The model under review builds one solid part; all positions refer to its coordinate system, in mm. Face numbers are marked on the shaded views. A direction names the side the tool comes from. Round coordinates to 2 decimals unless told otherwise and drop trailing zeros. Order: outer loops, then holes, each group sorted by start corner. A loop starts at its lowest first (then second) coordinate and runs counter-clockwise, first axis right, second up.
1) Consider section C-C (x = 391). Give the boundary of the cut face in (y, z), then the cut area to 3 significant figures.
2) Machinability: for the marked faces 4 and 5, which of the approach directions +Z, -Z, +X, -X, +Y, -Y give a long, thin tool a straight path to every point of the face, cutting with its end or side? Answer none if there is none.
3) To check wall thickness, follow L1, parallel to Y at x = 79, z = 375.5; L2, parallel to X at y = -32, z = 415; L3, parallel to Z at x = -2, y = -245. State the ranges of each line that lie inside material, in increasing order.
4) Clearance check with flat-ended pins moving along their axes: P1, Ø1.5, axis at x = -492.5, y = -59.5, coming from the +Z side; P2, Ø6, axis at y = -455, z = 342.5, coming from the -X side; P3, Ø5, axis at x = -239, y = -306.5, coming from the +Z side. State where each tip first meets the part, or that it passes through.
5) Consider section A-A (z = 413). Give the boundary of the cut face in (x, y).
6) Consider section B-B (y = -209.5). Give the boundary of the cut face in (x, z), then the cut area to 3 significant figures.
7) Consider section D-D (y = -528.5). Give the boundary of the cut face in (x, z).
8) Mouldability with a two-part tool opening along X and no side actions: class the marked faces 1, 2 and 3 as pulls with the +X half, pulls with the -X half, needs draft (parallel to the pull), parting line crosses it, or undercut.
from build123d import *

# Parameters (mm, degrees)
F0_W     = 1800
F0_H     = 800
F1_DEPTH = 440
F2_R     = 350
F4_DEPTH = 380
F5_R     = 200


with BuildPart() as f1:
    # F0 (on Top) → F1 (new body)
    with BuildSketch(Plane.XY):
        with Locations((-1.622595, -185.142654)):
            Rectangle(F0_W, F0_H)
    extrude(amount=F1_DEPTH)

    # F2
    f2_edges = [f1.edges().sort_by_distance(p)[0] for p in [
        (-901.622595, -585.142654, 220),
        (898.377405, -585.142654, 220),
    ]]
    fillet(f2_edges, radius=F2_R)

    # F3 (on face) → F4 (cut)
    with BuildSketch(Plane.XY.offset(440)):
        with BuildLine():
            Line((809.377417, 125.857358), (-812.622607, 125.857358))
            Line((-812.622607, 125.857358), (-812.622607, -235.142654))
            ThreePointArc((-812.622607, -235.142654), (-736.177473, -419.697533), (-551.622595, -496.142666))
            Line((-551.622595, -496.142666), (548.377405, -496.142666))
            ThreePointArc((548.377405, -496.142666), (732.932283, -419.697533), (809.377417, -235.142654))
            Line((809.377417, -235.142654), (809.377417, 125.857358))
        make_face()
    extrude(amount=-F4_DEPTH, mode=Mode.SUBTRACT)

    # F5
    f5_edges = [f1.edges().sort_by_distance(p)[0] for p in [
        (-812.622607, -54.642648, 60),
        (-736.177473, -419.697533, 60),
        (-1.622595, 125.857358, 60),
        (809.377417, -54.642648, 60),
        (732.932283, -419.697533, 60),
        (-1.622595, -496.142666, 60),
    ]]
    fillet(f5_edges, radius=F5_R)


solid = f1.part
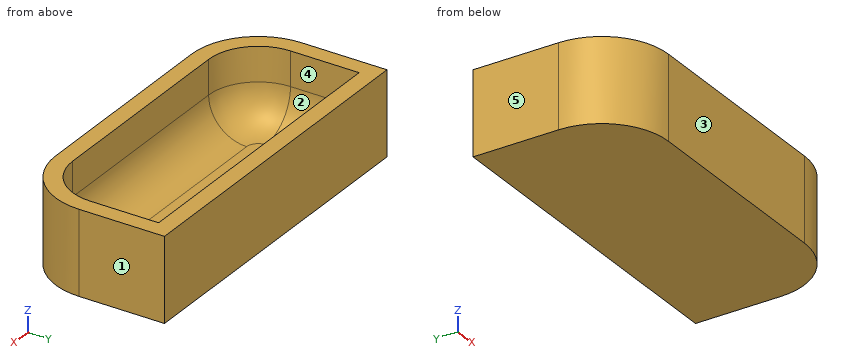
Answer below:
1. outline: (-585.14, 0) - (214.86, 0) - (214.86, 440) - (125.86, 440) - (125.86, 260) arc R200 cw to (-74.14, 60) - (-296.14, 60) arc R200 cw to (-496.14, 260) - (-496.14, 440) - (-585.14, 440) - close
1. area: 133,000 mm2
2. face 4: +Z
2. face 5: +Z, -Z, -X, +Y, -Y
3. L1: y = -585.14 to -496.14, 125.86 to 214.86
3. L2: x = -901.62 to -812.62, 809.38 to 898.38
3. L3: z = 0 to 60
4. P1: stops at z = 60.59
4. P2: stops at x = -826.35
4. P3: stops at z = 60.41
5. outline: (-901.62, -235.14) arc R350 ccw to (-551.62, -585.14) - (548.38, -585.14) arc R350 ccw to (898.38, -235.14) - (898.38, 214.86) - (-901.62, 214.86) - close; hole (-812.62, -235.14) arc R261 ccw to (-551.62, -496.14) - (548.38, -496.14) arc R261 ccw to (809.38, -235.14) - (809.38, 125.86) - (-812.62, 125.86) - close
6. outline: (-901.62, 0) - (898.38, 0) - (898.38, 440) - (809.38, 440) - (809.38, 260) arc R200 cw to (609.38, 60) - (-612.62, 60) arc R200 cw to (-812.62, 260) - (-812.62, 440) - (-901.62, 440) - close
6. area: 193,000 mm2
7. outline: (-742.52, 0) - (739.27, 0) - (739.27, 440) - (-742.52, 440) - close
8. face 1: pulls with the +X half
8. face 2: undercut
8. face 3: needs draft
